The listing builds one solid part. Answer for the finished solid, in the listing's coordinates (mm). Coordinates: 2 decimals unless noted, no trailing zeros. Return JSON: item names as keys, results as strings. Group by question number.
1. The mould has two halves that part along Z. Classify faces 1 (the face through (168, 5, -167)), 2 (the face through (332.576, 2.297, -26.34)): pulls with the +Z half, pulls with the -Z half, needs draft (parallel to the pull), parting line crosses it, or undercut.
2. Straight lines are drawn through the part: L1, parallel to Z at x = 264, y = 3.1; L2, parallel to X at y = 1.35, z = -35; L3, parallel to Z at x = 10, y = 3. For each, find the intervals that lie inside material, in ascending order. Write a range as from..to.
3. Given P1, Ø2, axis at x = 226, z = -47, coming from the -Y side, flat-ended and moving along its own axis, determine where the tip first touches the part or whether it passes through.
```python
from build123d import *

# Parameters (mm, degrees)
SKETCH_1_W                  = 340
SKETCH_1_H                  = 330
EXTRUDE_1_DEPTH             = 5
M4X0_7_2_D                  = 3.3
M4X0_7_2_DEPTH              = 11.5
M4X0_7_2_TIP                = 0.991420021
SKETCH_4_W                  = 1
SKETCH_4_H                  = 330
CUT_EXTRUDE_1_DEPTH         = 10
HOLE_WIZARD_M3_1_D          = 3.4
HOLE_WIZARD_M3_1_DEPTH      = 20
HOLE_WIZARD_M3_1_TIP        = 1.021463052
HOLE_WIZARD_M5_1_AT_2_COUNT = 2
HOLE_WIZARD_M5_1_AT_2_PITCH = 140
HOLE_WIZARD_M5_1_AT_3_COUNT = 2
HOLE_WIZARD_M5_1_AT_3_PITCH = 280
HOLE_WIZARD_M5_1_AT_4_COUNT = 2
HOLE_WIZARD_M5_1_AT_4_PITCH = 425.205832509
HOLE_WIZARD_M5_1_AT_5_COUNT = 2
HOLE_WIZARD_M5_1_AT_5_PITCH = 349.284983931
HOLE_WIZARD_M5_1_AT_6_COUNT = 2
HOLE_WIZARD_M5_1_AT_6_PITCH = 320


with BuildPart() as part:
    # 스케치1 → 보스-돌출1 (new body)
    with BuildSketch(Plane(origin=(0, 0, 0), x_dir=(1, 0, 0), z_dir=(0, 1, 0))):
        with Locations((170, 165)):
            Rectangle(SKETCH_1_W, SKETCH_1_H)
    extrude(amount=EXTRUDE_1_DEPTH)

    # M4x0.7 나사 구멍2
    with Locations(Plane(origin=(0, 5, 0), x_dir=(1, 0, 0), z_dir=(0, 1, 0))):
        with Locations((226, 281), (264, 281), (264, 35), (226, 35), (264, 47), (226, 47)):
            Hole(M4X0_7_2_D / 2, depth=M4X0_7_2_DEPTH)
            with Locations((0, 0, -(M4X0_7_2_DEPTH + M4X0_7_2_TIP / 2))):  # 118° drill point
                Cone(0, M4X0_7_2_D / 2, M4X0_7_2_TIP, mode=Mode.SUBTRACT)

    # 스케치4 → 컷-돌출1 (cut)
    with BuildSketch(Plane(origin=(0, 5, 0), x_dir=(1, 0, 0), z_dir=(0, 1, 0))):
        with Locations((339.5, 165)):
            Rectangle(SKETCH_4_W, SKETCH_4_H)
        with Locations((0.5, 165)):
            Rectangle(SKETCH_4_W, SKETCH_4_H)
    extrude(amount=-CUT_EXTRUDE_1_DEPTH, mode=Mode.SUBTRACT)

    # M3 여유 구멍1
    with Locations(Plane(origin=(0, 0, 0), x_dir=(-1, 0, 0), z_dir=(0, -1, 0))):
        with Locations((-199, 47), (-199, 87), (-199, 127), (-199, 167), (-199, 207), (-199, 247)):
            Hole(HOLE_WIZARD_M3_1_D / 2, depth=HOLE_WIZARD_M3_1_DEPTH)
            with Locations((0, 0, -(HOLE_WIZARD_M3_1_DEPTH + HOLE_WIZARD_M3_1_TIP / 2))):  # 118° drill point
                Cone(0, HOLE_WIZARD_M3_1_D / 2, HOLE_WIZARD_M3_1_TIP, mode=Mode.SUBTRACT)

    # 스케치7 → M5 납작 머리 작은 나사용 카운터싱크1 (revolve, cut)
    with BuildSketch(Plane(origin=(10, 0, -25), x_dir=(0, 0, -1), z_dir=(1, 0, 0))):
        Polygon((0, 0), (0, 5), (2.75, 5), (2.75, 2.45), (5.2, 0), align=None)
    hole_wizard_m5_1 = revolve(axis=Axis((10, -6.35, -25), (0, 1, 0)), mode=Mode.SUBTRACT)

    # M5 납작 머리 작은 나사용 카운터싱크1 at 2: M5 납작 머리 작은 나사용 카운터싱크1 ×2
    with Locations(*[(0, 0, -i * HOLE_WIZARD_M5_1_AT_2_PITCH) for i in range(1, HOLE_WIZARD_M5_1_AT_2_COUNT)]):
        add(hole_wizard_m5_1, mode=Mode.SUBTRACT)

    # M5 납작 머리 작은 나사용 카운터싱크1 at 3: M5 납작 머리 작은 나사용 카운터싱크1 ×2
    with Locations(*[(0, 0, -i * HOLE_WIZARD_M5_1_AT_3_PITCH) for i in range(1, HOLE_WIZARD_M5_1_AT_3_COUNT)]):
        add(hole_wizard_m5_1, mode=Mode.SUBTRACT)

    # M5 납작 머리 작은 나사용 카운터싱크1 at 4: M5 납작 머리 작은 나사용 카운터싱크1 ×2
    with Locations(*[Vector(0.7525766947068778, 0, -0.658504607868518) * (i * HOLE_WIZARD_M5_1_AT_4_PITCH) for i in range(1, HOLE_WIZARD_M5_1_AT_4_COUNT)]):
        add(hole_wizard_m5_1, mode=Mode.SUBTRACT)

    # M5 납작 머리 작은 나사용 카운터싱크1 at 5: M5 납작 머리 작은 나사용 카운터싱크1 ×2
    with Locations(*[Vector(0.9161573349021892, 0, -0.4008188340197077) * (i * HOLE_WIZARD_M5_1_AT_5_PITCH) for i in range(1, HOLE_WIZARD_M5_1_AT_5_COUNT)]):
        add(hole_wizard_m5_1, mode=Mode.SUBTRACT)

    # M5 납작 머리 작은 나사용 카운터싱크1 at 6: M5 납작 머리 작은 나사용 카운터싱크1 ×2
    with Locations(*[(i * HOLE_WIZARD_M5_1_AT_6_PITCH, 0, 0) for i in range(1, HOLE_WIZARD_M5_1_AT_6_COUNT)]):
        add(hole_wizard_m5_1, mode=Mode.SUBTRACT)


solid = part.part
```
Worked out:
{
 "1": {"face 1": "needs draft", "face 2": "undercut"},
 "2": {"L1": "-330..-282.65, -279.35..-48.65, -45.35..-36.65, -33.35..0", "L2": "1..224.35, 227.65..262.35, 265.65..339", "L3": "-330..-307.75, -302.25..-167.75, -162.25..-27.75, -22.25..0"},
 "3": {"P1": "through"}
}
